Input: dimensioned drawing with shaded views. Units: mm. Origin: part minimum x, y, z. A direction names the side the tool comes from. Give positions to 0.01 mm unless a question says otherwise; leave off trailing zeros. Write each loop counter-clockwise with the first axis right and the second up, starting at its lowest first coordinate (ties: lowest second). Pieces come first, ordered by that corner, then holes. Notation, with made-up numbers: (78.25, 88.5) -> (92.25, 88.5) arc R25 cw to (92.25, 103.5) -> close; hole circle Ø6 at (-28, -33). An arc over 180 degrees is marked (long way). Answer as a JSON object with one key per item and string values.
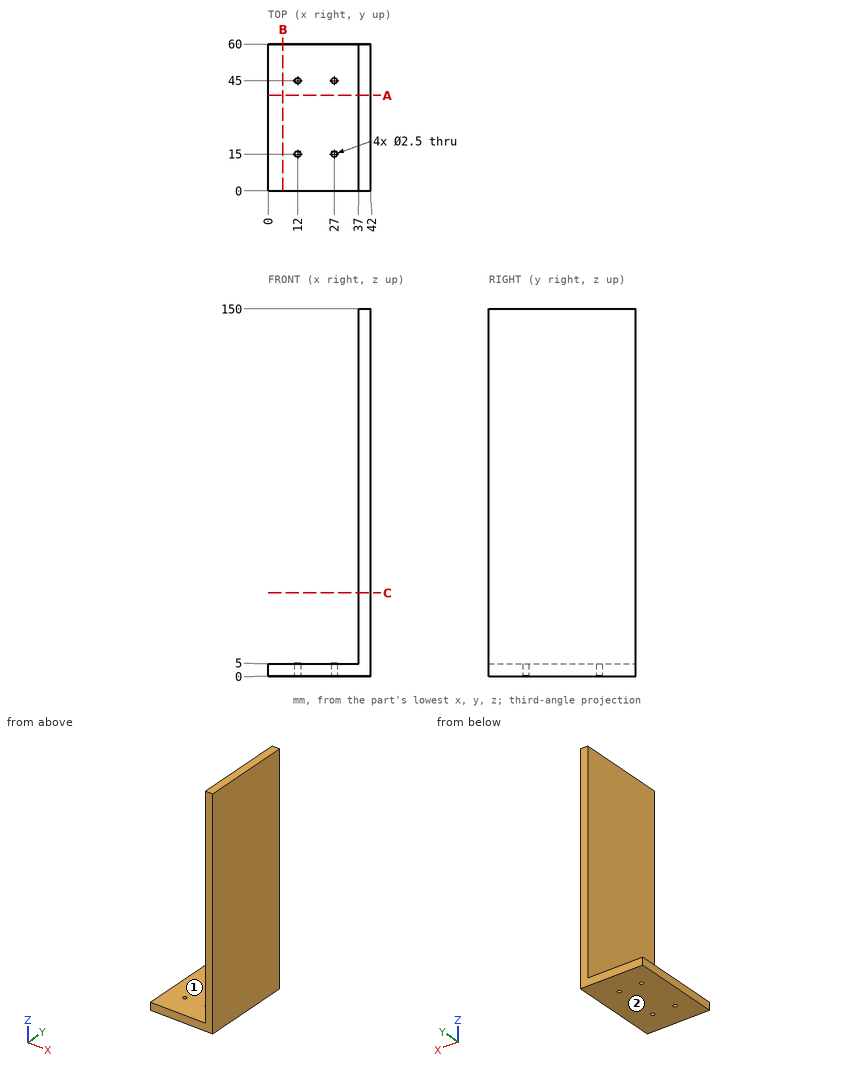
Q1. Cut plane B-B (x = 6). Return the cut outline in (y, z), and give its area (3 significant figures).
Values:
{"outline": "(0, 0) -> (60, 0) -> (60, 5) -> (0, 5) -> close", "area": "300 mm²"}
Q2. Cut plane A-A (y = 39). Return the cut outline in (x, z), and give its area (3 significant figures).
Values:
{"outline": "(0, 0) -> (42, 0) -> (42, 150) -> (37, 150) -> (37, 5) -> (0, 5) -> close", "area": "935 mm²"}
Q3. Cut plane C-C (z = 34). Return the cut outline in (x, y), and give its area (3 significant figures).
Values:
{"outline": "(37, 0) -> (42, 0) -> (42, 60) -> (37, 60) -> close", "area": "300 mm²"}
Q4. Material intervals for L1, parallel to Y at x = 12, z = 1.1; L2, parallel to X at y = 56.5, z = 43; L3, parallel to Z at x = 2, y = 36.5, sorted ascending. Write a range as from..to.
Values:
{"L1": "0..13.75, 16.25..43.75, 46.25..60", "L2": "37..42", "L3": "0..5"}
Q5. First-contact query: P1, Ø3, axis at x = 27, y = 15, coming from the +Z side; P2, Ø12, axis at y = 44, z = 84, coming from the -X side. Flat tips, straight axial feed; report the tip coordinate or a pass-through.
Values:
{"P1": "z = 5", "P2": "x = 37"}
Q6. Set-up query: the marked faces 1 and 2. Return all of +Z, -Z, +X, -X, +Y, -Y with unobstructed straight access to the full face (end or side cutting, diameter ignored); none if empty.
Values:
{"face 1": "+Z, -X, +Y, -Y", "face 2": "-Z, +X, -X, +Y, -Y"}
